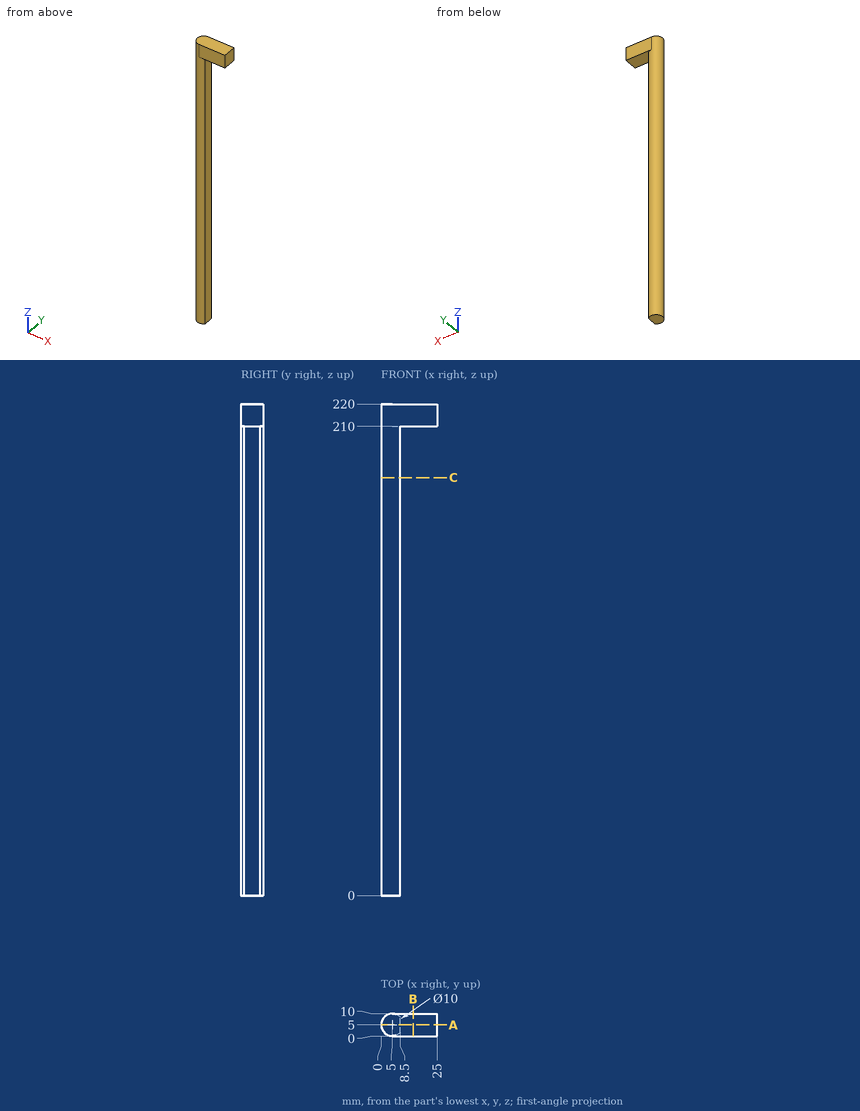
Verification items for this drawing (mm, ordinates from the low corner). Give positions to 0.01 mm unless a question says otherwise; leave off trailing zeros. Loops run counter-clockwise (first coordinate to the right, second up) from the corner with the lowest first, then second, coordinate; pieces in that order, holes last.
1. Cross-section at C-C on z = 187. Record the cut outline in (x, y).
Derived:
outline: (8.5, 1.43) - (8.5, 8.57) arc R5 ccw (long way) to start
2. Material ranges on probe 1 along X at (y, z) = (1.5, 100); probe 2 along X at (y, z) = (5.5, 194); probe 3 along Z at (x, y) = (11.5, 9), recorded low to high.
Derived:
probe 1: x = 1.43 to 8.5
probe 2: x = 0.03 to 8.5
probe 3: z = 210 to 220
3. Go/stop test with flat-tipped pins: P1, Ø1, axis at y = 7.5, z = 123.5, coming from the +X side; P2, Ø1, axis at x = 6.5, z = 63, coming from the +Y side; P3, Ø5, axis at x = 9.5, z = 194.5, coming from the -Y side. Record where each tip stops, or that it passes through.
Derived:
P1: stops at x = 8.5
P2: stops at y = 9.9
P3: stops at y = 0.42
4. Cross-section at B-B on x = 14.25. Record the cut outline in (y, z).
Derived:
outline: (0, 210) - (10, 210) - (10, 220) - (0, 220) - close
5. Cross-section at A-A on y = 5. Record the cut outline in (x, z), and give its area (4 significant figures).
Derived:
outline: (0, 0) - (8.5, 0) - (8.5, 210) - (25, 210) - (25, 220) - (0, 220) - close
area: 2,035 mm2
